Geometry check sheet. Reference: the model listing, model coordinates, mm. Coordinates: 2 decimals unless noted, no trailing zeros. Write each loop counter-clockwise with the first axis right and the second up, starting at its lowest first coordinate (ties: lowest second). Pieces come first, ordered by that corner, then holes. Notation, with made-up numbers: (-38, 20.25) -> (-26, 20.25) arc R24 cw to (-26, 53.25) -> close; hole circle Ø9 at (13, 13). An arc over 180 degrees is marked (long way). Answer in a Markdown table with one row per item. Add a question column.
Q1. Section check A-A, the plane z = 5. Record the boundary of the cut face in (x, y), and give its area (3 significant figures).
Q2. Section check B-B, the plane y = 7. Record the boundary of the cut face in (x, z).
Q3. Gauge pin test, flat ends, axial feed: P1, Ø4.5, axis at y = 27, z = 0, coming from the -X side; P2, Ø6.5, axis at x = 0, y = 293, coming from the +Z side. Record the tip position at first contact, or that the pin passes through.
Q4. Section check D-D, the plane y = 176. Record the boundary of the cut face in (x, z), and give its area (3 significant figures).
Q5. Thickness scan on line 1 (Y direction, x = 0, z = 8.6); line 2 (X direction, y = 273, z = 8.6); line 3 (X direction, y = 261.5, z = 0.25). Record the ranges inside material, lowest first.
Q6. Section check C-C, the plane x = 5.25. Record the boundary of the cut face in (y, z).
```python
from build123d import *

# Parameters (mm, degrees)
F1_W       = 19
F1_H       = 19
F1_W_2     = 16.6
F1_H_2     = 16.6
F2_DEPTH   = 300
F5_D       = 5
F5_ON_F4_D = 5


# Not quite as in the source:
# - a feature names something its author has since deleted; it is built from what else it names


with BuildPart() as f2:
    # F1 (on Front) → F2 (new body)
    with BuildSketch(Plane.XZ):
        Rectangle(F1_W, F1_H)
        Rectangle(F1_W_2, F1_H_2, mode=Mode.SUBTRACT)
    extrude(amount=-F2_DEPTH)

    # F5 (through all)
    with Locations(Plane.YZ.offset(9.5)):
        with Locations((7, 0), (27, 0)):
            Hole(F5_D / 2)

    # F5 on F4 (through all)
    with Locations(Plane.XY.offset(9.5)):
        with Locations((0, 273), (0, 293)):
            Hole(F5_ON_F4_D / 2)


solid = f2.part
```
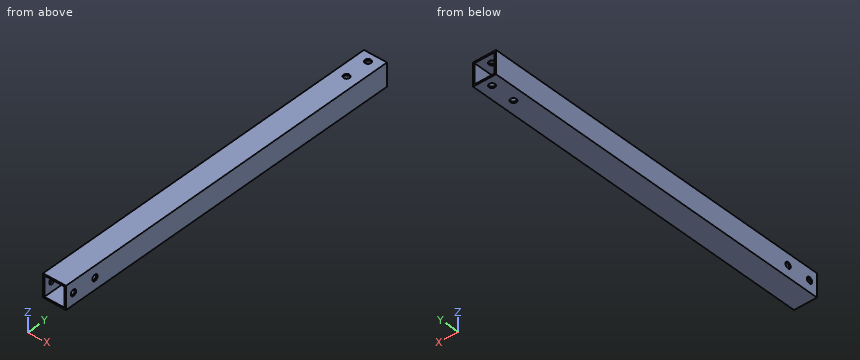
Calculated:
| question | item | result |
|---|---|---|
| 1 | outline | (-9.5, 0) -> (-8.3, 0) -> (-8.3, 300) -> (-9.5, 300) -> close; (8.3, 0) -> (9.5, 0) -> (9.5, 300) -> (8.3, 300) -> close |
| 1 | area | 720 mm² |
| 2 | outline | (-9.5, -9.5) -> (9.5, -9.5) -> (9.5, -2.5) -> (8.3, -2.5) -> (8.3, -8.3) -> (-8.3, -8.3) -> (-8.3, -2.5) -> (-9.5, -2.5) -> close; (-9.5, 2.5) -> (-8.3, 2.5) -> (-8.3, 8.3) -> (8.3, 8.3) -> (8.3, 2.5) -> (9.5, 2.5) -> (9.5, 9.5) -> (-9.5, 9.5) -> close |
| 3 | P1 | passes through |
| 3 | P2 | stops at z = 9.5 |
| 4 | outline | (-9.5, -9.5) -> (9.5, -9.5) -> (9.5, 9.5) -> (-9.5, 9.5) -> close; hole (-8.3, -8.3) -> (8.3, -8.3) -> (8.3, 8.3) -> (-8.3, 8.3) -> close |
| 4 | area | 85.4 mm² |
| 5 | line 1 | y = 0 to 270.5, 275.5 to 290.5, 295.5 to 300 |
| 5 | line 2 | x = -9.5 to -2.5, 2.5 to 9.5 |
| 5 | line 3 | x = -9.5 to -8.3, 8.3 to 9.5 |
| 6 | outline | (0, -9.5) -> (300, -9.5) -> (300, -8.3) -> (0, -8.3) -> close; (0, 8.3) -> (300, 8.3) -> (300, 9.5) -> (0, 9.5) -> close |
